Read the model definition and answer for the solid it produces. Units are mm, in the model's axes. Face numbers are marked on the shaded views. A direction names the side the tool comes from. Round coordinates to 2 decimals unless told otherwise and drop trailing zeros. Write each loop counter-clockwise with the first axis right and the second up, starting at its lowest first coordinate (ties: lowest second). Pieces come first, ordered by that corner, then holes. Notation, with made-up numbers: (56, 68.5) - (78, 68.5) arc R17 cw to (78, 75.5) - close; hole circle Ø9 at (-13.75, 83). An arc over 180 degrees is marked (long way). Answer as CSV lines item,"result". Start each with the question number.
1) Find section B-B on x = -93.5. Determine the outline of the cut face in (y, z), then the cut area to 3 significant figures.
2) Find section A-A on z = 0. Determine the outline of the cut face in (x, y).
3) Which of the six approach directions +Z, -Z, +X, -X, +Y, -Y give full straight-line access (tool end or side, diameter ignored) to the marked faces 1 and 2?
4) Each of these flat-tipped pins is pushed along its axis until it touches: pin 1 (8 mm diameter, centred on x = -60, z = -2.5, fed in from +Y); pin 2 (1 mm diameter, centred on y = 6, z = 10.5, fed in from -X); pin 3 (10 mm diameter, centred on x = -13, y = -9.5, fed in from +Z). Where does it stop, or does it pass through?
5) Consider line 1 along X through (y, z) = (0, -2); line 2 along X through (y, z) = (-9.5, 6); line 3 along X through (y, z) = (-0.5, -6.5). Determine where each line is inside the solid, lowest interval first.
Autodesk Inventor part; units mm, degrees
ref_plane "YZ Plane" through (0, 0, 0) normal (1, 0, 0) x (0, 1, 0)
ref_plane "XZ Plane" through (0, 0, 0) normal (0, 1, 0) x (-1, 0, 0)
ref_plane "XY Plane" through (0, 0, 0) normal (0, 0, 1) x (1, 0, 0)
sketch "Sketch1" plane through (0, 0, 0) normal (0, 0, 1) x (1, 0, 0)
  line L0 (-148.0565, 0) -> (148.0565, 0)
  line L1 (-148.0565, 0) -> (-148.0565, 8)
  line L2 (-148.0565, 8) -> (143.0565, 8)
  line L3 (143.0565, 8) -> (143.0565, 15)
  line L4 (143.0565, 15) -> (148.0565, 15)
  line L5 (148.0565, 15) -> (148.0565, 0)
  circle A0 centre (-143.0565, 0) radius 1.75
  point P0 (0, 0)
  point P1 (0, 0)
  point P2 (143.0565, 8.25)
  dimension "d0" = 296.113
  dimension "d1" = 16
  dimension "d2" = 5
  dimension "d3" = 30
  dimension "d8" = 3.5
  dimension "d9" = 5
  dimension "d12" = 0.25
revolve "Revolution1" add sketch "Sketch1" angle 360 about axis through (-148.0565, 0, 0) along (1, 0, 0) picked at (-142.9862, 0.5791) contours A0 L0 L1 L2 L3 L4 L5 | L0 A0
fillet "Fillet1" radius 1 1 edges at (-148.0565, -8, 0)
chamfer "Chamfer1" distance 1 angle 45 3 edges at (148.0565, -15, 0) (-147.0565, -8, 0) (-148.0565, -7, 0)
extrude "Extrusion2" cut sketch "Sketch1" against normal through all both and the other way through all contours A0 L0 | L0 A0
properties part number "PWTR-0137" material "Stainless Steel"
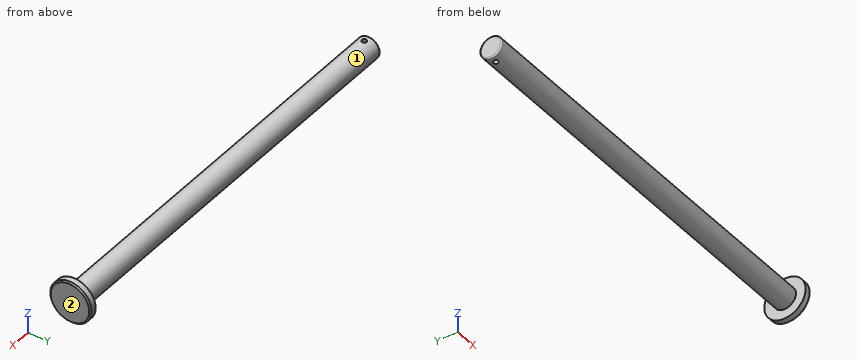
Check values:
1,outline,"circle Ø16 at (0, 0)"
1,area,"201 mm^2"
2,outline,"(-148.06, -7) arc R1 ccw to (-147.06, -8) - (143.06, -8) - (143.06, -15) - (147.06, -15) - (148.06, -14) - (148.06, 14) - (147.06, 15) - (143.06, 15) - (143.06, 8) - (-147.06, 8) arc R1 ccw to (-148.06, 7) - close; hole circle Ø3.5 at (-143.06, 0)"
3,face 1,"-X"
3,face 2,"+Z, -Z, +X, +Y, -Y"
4,pin 1,"stops at y = 8"
4,pin 2,"stops at x = 143.06"
4,pin 3,"stops at z = 6.61"
5,line 1,"x = -148.06 to -144.81, -141.31 to 148.06"
5,line 2,"x = 143.06 to 148.06"
5,line 3,"x = -148.06 to -144.73, -141.38 to 148.06"
